The drawing under review shows one solid part. Ordinate dimensions are in mm from its lowest x, y, z. A direction names the side the tool comes from. Coordinates: 2 decimals unless noted, no trailing zeros. Loops run counter-clockwise (first coordinate to the right, second up) from the corner with the lowest first, then second, coordinate; pieces in that order, holes last. Notation, with made-up numbers: M 84.25,-19.75 L 101.25,-19.75 A11 cw 101.25,-3.75 Z; hole C 61,71 d2. An arc over 180 degrees is marked long. Use one line per item in the form item = value.
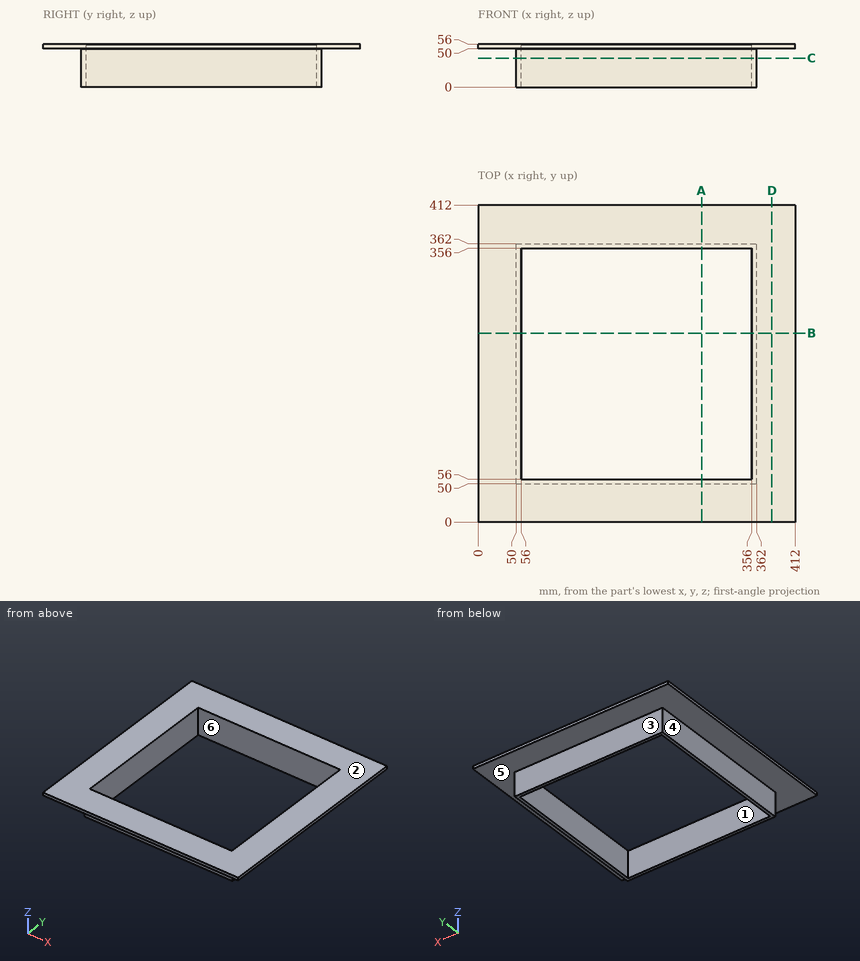
1. For pin 1 Ø4 at (x, z) = (156.5, 25.5) entering from +Y; pin 2 Ø15 at (y, z) = (199, 24) entering from -X; pin 3 Ø8 at (x, z) = (130.5, 33.5) entering from -Y, all flat-tipped, find the tip position at first contact; note any pin that passes through.
Computed values:
pin_1 = 362
pin_2 = 50
pin_3 = 50
2. Consider section A-A on x = 290.5. Write out the cut boundary in (y, z).
Computed values:
outline = M 0,50 L 50,50 L 50,0 L 56,0 L 56,56 L 0,56 Z; M 356,0 L 362,0 L 362,50 L 412,50 L 412,56 L 356,56 Z
3. Consider section C-C on z = 37.5. Write out the cut boundary in (x, y).
Computed values:
outline = M 50,50 L 362,50 L 362,362 L 50,362 Z; hole M 56,56 L 356,56 L 356,356 L 56,356 Z
4. Tool access review of the marked faces 1, 2 and 3: name each direction out of +Z, -Z, +X, -X, +Y, -Y from which nothing blocks a thin tool from reaching the whole face with its end or side.
Computed values:
face_1 = +Z, -Z
face_2 = +Z, +X, -X, +Y, -Y
face_3 = -Z, +X, -X, +Y
5. Consider section D-D on x = 382. Write out the cut boundary in (y, z), plus the area to 3 significant figures.
Computed values:
outline = M 0,50 L 412,50 L 412,56 L 0,56 Z
area = 2,470 mm2
6. Wall thickness on line 1 along Y through (x, z) = (352, 15); line 2 along Y through (x, z) = (220, 53.5): over which ranges is each line inside the solid? List them lowest first. Write a range as from..to.
Computed values:
line_1 = 50..56, 356..362
line_2 = 0..56, 356..412
7. Draft analysis for pull direction X (two halves, no side actions). For the marked faces 4, 5 and 6, state which applies: +X half, -X half, draft (parallel to the pull), parting line (faces both ways), or undercut.
Computed values:
face_4 = -X half
face_5 = draft
face_6 = undercut
